Job drawing, mm, ordinate dimensions from the low corner. One solid piece. Round coordinates to 2 decimals unless told otherwise and drop trailing zeros. Order: outer loops, then holes, each group sorted by start corner. A loop starts at its lowest first (then second) coordinate and runs counter-clockwise, first axis right, second up. Notation, with made-up numbers: (7, 73.5) - (46, 73.5) arc R25 ccw to (46, 93.5) - close; hole circle Ø4 at (86, 59.5). An arc over 180 degrees is marked (long way). Use one line per item in the form item = value. Start each with the question number.
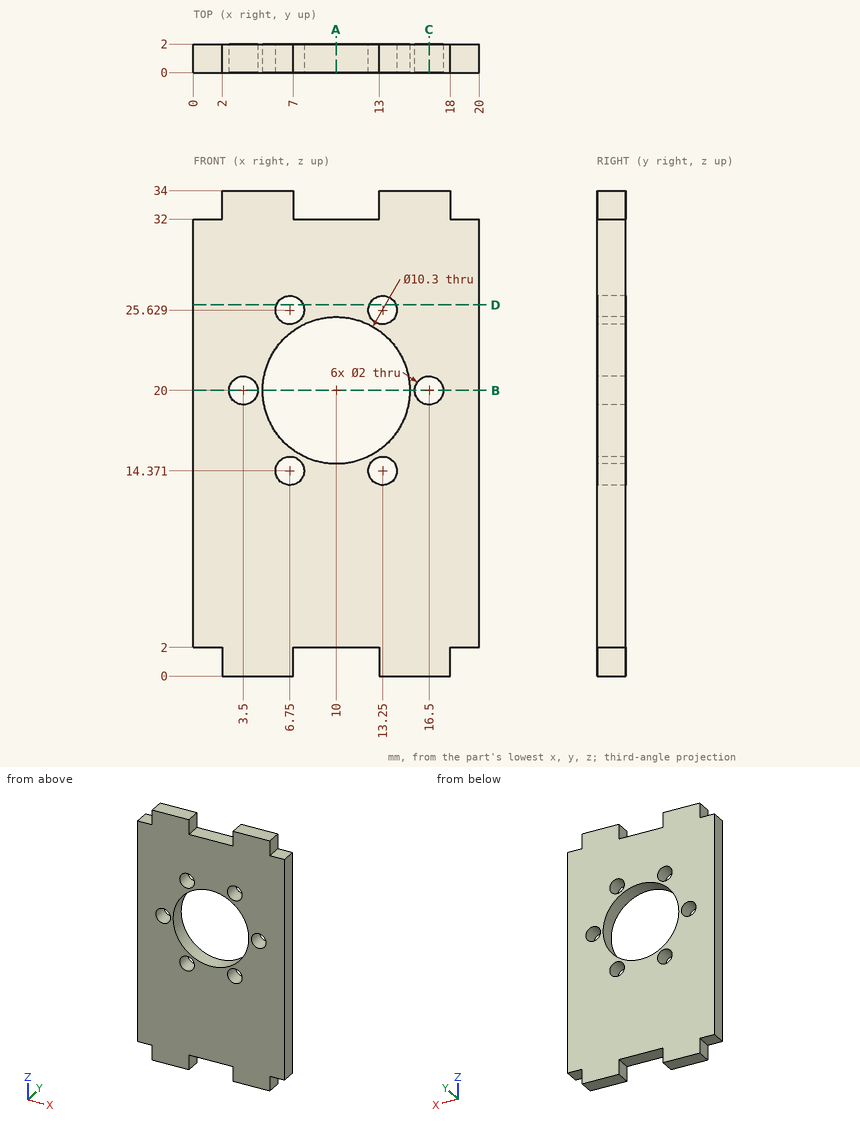
(1) Slice it at D-D (z = 26). Give the cut face in (x, y), and give its area (3 significant figures).
(2) Slice it at B-B (z = 20). Give the cut face in (x, y).
(3) Slice it at A-A (x = 10). Give the cut face in (y, z).
(4) Wall check: line 1 (Z direction, x = 3.5, y = 0.45); line 2 (Z direction, x = 10, y = 0.6); line 3 (Z direction, x = 12.75, y = 0.7) (1 decimal). Give the ranges that are in metal, low to high. Write a range as [from, to].
(5) Flat gauge pins, fed straight in: P1, Ø0.6, axis at y = 0.5, z = 1, coming from the +X side; P2, Ø1.6, axis at x = 6.75, z = 14.37, coming from the +Y side. Where does each tip first touch, or does it go through?
(6) Slice it at C-C (x = 16.5). Give the cut face in (y, z), and give its area (3 significant figures).
Results list:
q1.outline = (0, 0) - (5.82, 0) - (5.82, 2) - (0, 2) - close; (7.68, 0) - (12.32, 0) - (12.32, 2) - (7.68, 2) - close; (14.18, 0) - (20, 0) - (20, 2) - (14.18, 2) - close
q1.area = 32.6 mm²
q2.outline = (0, 0) - (2.5, 0) - (2.5, 2) - (0, 2) - close; (4.5, 0) - (4.85, 0) - (4.85, 2) - (4.5, 2) - close; (15.15, 0) - (15.5, 0) - (15.5, 2) - (15.15, 2) - close; (17.5, 0) - (20, 0) - (20, 2) - (17.5, 2) - close
q3.outline = (0, 2) - (2, 2) - (2, 14.85) - (0, 14.85) - close; (0, 25.15) - (2, 25.15) - (2, 32) - (0, 32) - close
q4.line_1 = [0, 19], [21, 34]
q4.line_2 = [2, 14.85], [25.15, 32]
q4.line_3 = [2, 13.5], [15.2, 15.6], [24.4, 24.8], [26.5, 32]
q5.P1 = 18
q5.P2 = through
q6.outline = (0, 0) - (2, 0) - (2, 19) - (0, 19) - close; (0, 21) - (2, 21) - (2, 34) - (0, 34) - close
q6.area = 64.0 mm²
